Can you work these out from the model? Positions are in its coordinate system, mm. Give positions to 0.01 mm unless a question says otherwise; leave off trailing zeros. Write each loop counter-clockwise with the first axis right and the second up, starting at its lowest first coordinate (ties: lowest second). Pieces come first, ordered by that corner, then holes. Notation, with made-up numbers: M 35.5,-29 L 80.5,-29 A23 cw 80.5,4 Z; hole C -18,39.5 d2. An arc over 180 degrees is marked long. Use CSV: the item, a comma, the result in double quotes. Start each with the question number.
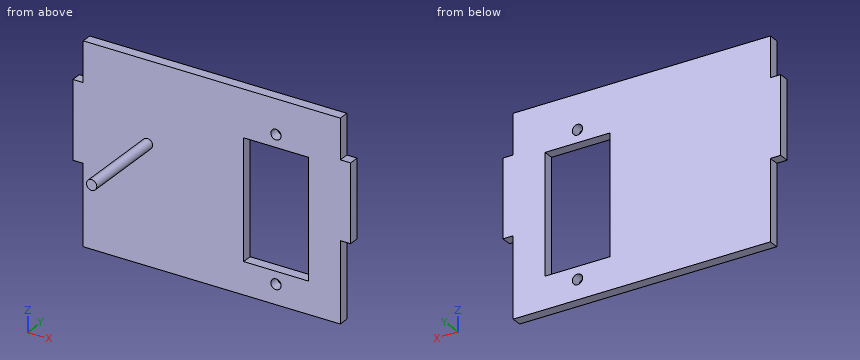
from build123d import *

# Parameters (mm, degrees)
SKETCH1_R           = 1
BOSS_EXTRUDE1_DEPTH = 2
SKETCH2_R           = 1
BOSS_EXTRUDE2_DEPTH = 17
SKETCH3_W           = 50
SKETCH3_H           = 7.75
CUT_EXTRUDE1_DEPTH  = 2


with BuildPart() as part:
    # Sketch1 → Boss-Extrude1 (new body)
    with BuildSketch(Plane(origin=(0, 0, 0), x_dir=(1, 0, 0), z_dir=(0, 1, 0))):
        Polygon((-25, 23), (25, 23), (25, 7.5), (27, 7.5), (27, -7.5), (25, -7.5), (25, -23), (-25, -23), (-25, -7.5), (-27, -7.5), (-27, 7.5), (-25, 7.5), align=None)
        with Locations(Location((12.5, 19.2, 0), (0, 0, 270))):
            Circle(SKETCH1_R, mode=Mode.SUBTRACT)
        with Locations(Location((12.5, -8.6, 0), (0, 0, 90))):
            Circle(SKETCH1_R, mode=Mode.SUBTRACT)
        Polygon((6.2, 16.8), (6.2, 6.2), (6.2, -6.2), (18.8, -6.2), (18.8, 6.2), (18.8, 16.8), align=None, mode=Mode.SUBTRACT)
    extrude(amount=BOSS_EXTRUDE1_DEPTH)

    # Sketch2 → Boss-Extrude2 (add)
    with BuildSketch(Plane.XZ):
        with Locations(Location((-12.5, -0.300349058, 0), (0, 0, 90))):
            Circle(SKETCH2_R)
    extrude(amount=BOSS_EXTRUDE2_DEPTH)

    # Sketch3 → Cut-Extrude1 (cut)
    with BuildSketch(Plane.XZ):
        with Locations((0, 19.125)):
            Rectangle(SKETCH3_W, SKETCH3_H)
    extrude(amount=-CUT_EXTRUDE1_DEPTH, mode=Mode.SUBTRACT)


solid = part.part
(1) Please list where these lines run through material, in increasing order: L1, parallel to X at y = 0.75, z = -19.2; L2, parallel to Y at x = -5, z = 12.5; L3, parallel to Z at x = 15, y = 0.5. Write a range as [from, to].
(2) Will these pins go through, and if not, where does the flat tip stop? pin 1 Ø1.6 at (x, z) = (12.5, -19.2) entering from +Y; pin 2 Ø0.6 at (y, z) = (1, 10) entering from -X; pin 3 Ø1 at (y, z) = (0.5, -18) entering from +X; pin 4 Ø1.6 at (x, y) = (-26, 0.5) entering from -Z.
(3) I want a section at D-D (y = -12.5). Write out the boundary of the cut face in (x, z), and give its area (3 significant figures).
(4) I want a section at C-C (x = -12.5). Write out the boundary of the cut face in (y, z).
(5) I want a section at B-B (x = 15.5). Write out the boundary of the cut face in (y, z).
(6) I want a section at A-A (z = -11). Write out the boundary of the cut face in (x, y).
Geometry results:
1,L1,"x = [-25, 11.5], [13.5, 25]"
1,L2,"y = [0, 2]"
1,L3,"z = [-23, -16.8], [6.2, 15.25]"
2,pin 1,"passes through"
2,pin 2,"stops at x = -25"
2,pin 3,"stops at x = 25"
2,pin 4,"stops at z = -7.5"
3,outline,"C -12.5,-0.3 d2"
3,area,"3.14 mm2"
4,outline,"M -17,-1.3 L 0,-1.3 L 0,-23 L 2,-23 L 2,15.25 L 0,15.25 L 0,0.7 L -17,0.7 Z"
5,outline,"M 0,-23 L 2,-23 L 2,-16.8 L 0,-16.8 Z; M 0,6.2 L 2,6.2 L 2,15.25 L 0,15.25 Z"
6,outline,"M -25,0 L 6.2,0 L 6.2,2 L -25,2 Z; M 18.8,0 L 25,0 L 25,2 L 18.8,2 Z"
